Input: part model. Units: mm. Frame: model coordinates. A direction names the side the tool comes from. Coordinates: 2 decimals unless noted, no trailing zeros. Write each loop counter-clockwise with the first axis right and the second up, starting at its lowest first coordinate (ties: lowest second). Pieces come first, ordered by that corner, then holes.
from build123d import *

# Parameters (mm, degrees)
BASENUT_DEPTH     = 17.8
SKETCH3_R         = 5.5
HOLE_DEPTH        = 28.12289531
SLOT_DEPTH        = 37.36697762
SLOTPATTERN_COUNT = 6


with BuildPart() as part:
    # Sketch1 → BaseNut (new body)
    with BuildSketch(Plane.XY):
        Polygon((6.062177826, -10.5), (12.124355653, 0), (6.062177826, 10.5), (-6.062177826, 10.5), (-12.124355653, 0), (-6.062177826, -10.5), align=None)
    extrude(amount=-BASENUT_DEPTH)

    # Sketch2 → Double-Chamfer (revolve, cut)
    with BuildSketch(Plane(origin=(-3.47179677, 0, -17.32820323), x_dir=(0, 0, -1), z_dir=(0, 1, 0))):
        Polygon((0.47179677, 6.32820323), (-0.374199502, 8.652558883), (0.47179677, 8.652558883), align=None)
        Polygon((-17.32820323, 6.32820323), (-17.32820323, 8.652558883), (-16.482206959, 8.652558883), align=None)
    revolve(axis=Axis((0, 0, -17.32820323), (0, 0, 1)), mode=Mode.SUBTRACT)

    # Sketch3 → Hole (cut, through all)
    with BuildSketch(Plane(origin=(-4.279914938, -1.735659213, -17.8), x_dir=(-1, 0, 0), z_dir=(0, 0, -1))):
        with Locations((-4.279914938, 1.735659213)):
            Circle(SKETCH3_R)
    extrude(amount=-HOLE_DEPTH, mode=Mode.SUBTRACT)

    # Sketch4 → EndChamfer (revolve, cut)
    with BuildSketch(Plane(origin=(-15.758283222, 0, -7.108283222), x_dir=(0, 0, -1), z_dir=(0, 1, 0)), mode=Mode.PRIVATE) as endchamfer_sk:
        Polygon((10.691716778, -23.308283222), (8.641716778, -21.258283222), (10.691716778, -21.258283222), align=None)
        Polygon((-7.108283222, -21.258283222), (-5.058283222, -21.258283222), (-7.108283222, -23.308283222), align=None)
    revolve(endchamfer_sk.sketch.rotate(Axis((0, 0, -7.108283222), (0, 0, 1)), 180), axis=Axis((0, 0, -7.108283222), (0, 0, 1)), mode=Mode.SUBTRACT)

    # Sketch5 → Slot (cut, through all)
    with BuildSketch(Plane(origin=(-17.8, 0, -17.8), x_dir=(0, 0, -1), z_dir=(0, 1, 0))):
        with BuildLine():
            Line((-17.8, -15.675), (-14.925, -15.675))
            ThreePointArc((-14.925, -15.675), (-12.8, -17.8), (-14.925, -19.925))
            Line((-14.925, -19.925), (-17.8, -19.925))
            Line((-17.8, -19.925), (-17.8, -15.675))
        make_face()
    slot = extrude(amount=-SLOT_DEPTH, mode=Mode.SUBTRACT)

    # SlotPattern: Slot ×6 about axis
    slotpattern_axis = Axis((0, 0, 0), (0, 0, 1))
    for i in range(1, SLOTPATTERN_COUNT):
        add(slot.rotate(slotpattern_axis, i * 360 / SLOTPATTERN_COUNT), mode=Mode.SUBTRACT)


solid = part.part
Item 1: Section query B-B, the plane x = 0. Return loops of the section in (y, z).
Item 2: Section query A-A, the plane z = -5.75. Return loops of the section in (x, y).
Item 3: Pin query (flat end, axial travel): pin 1 Ø3 at (y, z) = (-9, -1) entering from -X; pin 2 Ø3 at (y, z) = (4.5, -5) entering from +X; pin 3 Ø2.5 at (y, z) = (6.5, -2) entering from -X. Return the tip coordinate at first contact, or that it passes through.
Item 4: Material intervals for line 1 (Y direction, x = 0, z = -5.25); line 2 (Y direction, x = -6, z = -3); line 3 (X direction, y = -1, z = -16), sorted ascending.
Item 5: Access query for faces 1 (the face through (-8.3, -2.34, -1.42)), 2 (the face through (0, 8, -5)). Directions: +Z, -Z, +X, -X, +Y, -Y. A direction counts if a zero-diameter tool reaches every point of the face in a straight line with its end or side. Return the directions, or none.
Item 6: Pull-direction query (X, two-part tool) for faces 3 (the face through (3.251, -5.674, -1.011)), 4 (the face through (4, 8, 0)), 5 (the face through (-10.43, 0.05, -0.23)), 6 (the face through (5.17, -9.06, -0.23)); classes: released by +X, released by -X, zero draft, split by the parting line, or undercut.
The answers:
1. outline: (-10.5, -17.55) - (-9.8, -17.8) - (-7.55, -17.8) - (-5.5, -15.75) - (-5.5, -5) - (-10.5, -5) - close; (5.5, -15.75) - (7.55, -17.8) - (9.8, -17.8) - (10.5, -17.55) - (10.5, -5) - (5.5, -5) - close
2. outline: (-12.12, 0) - (-6.06, -10.5) - (6.06, -10.5) - (12.12, 0) - (6.06, 10.5) - (-6.06, 10.5) - close; hole circle Ø11 at (0, 0)
3. pin 1: stops at x = -7.79
3. pin 2: stops at x = 10.39
3. pin 3: stops at x = -8.04
4. line 1: y = -10.5 to -5.5, 5.5 to 10.5
4. line 2: y = -10.5 to -5.91, -1.01 to 1.01, 5.91 to 10.5
4. line 3: x = -11.55 to -5.66, 5.66 to 11.55
5. face 1: +Z
5. face 2: +Z, +Y, -Y
6. face 3: undercut
6. face 4: zero draft
6. face 5: released by -X
6. face 6: released by +X
